Check sheet for the modelled part. Datum: model origin and axes. Units: mm. Face numbers are marked on the shaded views. A direction names the side the tool comes from. Give positions to 0.01 mm unless a question says otherwise; leave off trailing zeros. Order: outer loops, then holes, each group sorted by start corner. A loop starts at its lowest first (then second) coordinate and runs counter-clockwise, first axis right, second up.
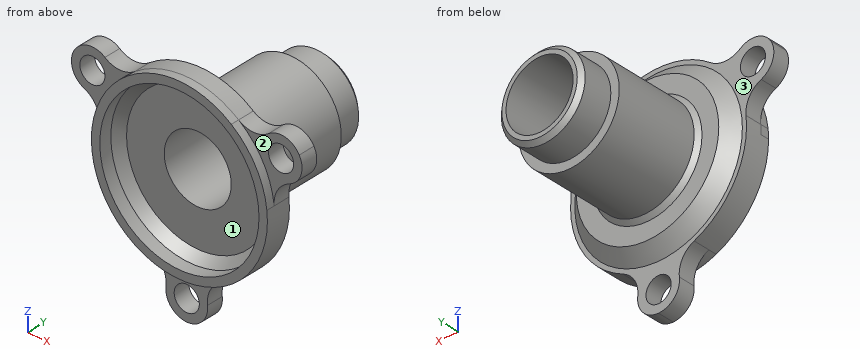
```python
from build123d import *

# Parameters (mm, degrees)
CHAMFER_1_SIZE      = 0.5
SKETCH_2_R          = 1.5
CUT_EXTRUDE_1_DEPTH = 28.256925725


with BuildPart() as part:
    # 草图1 → 旋转1 (revolve)
    with BuildSketch(Plane.XY, mode=Mode.PRIVATE) as revolve_1_sk:
        Polygon((10.5, 0), (15.5, 0), (15.5, 2), (10, 2), (8.5, 3.5), (6, 3.5), (6, 14.2), (5, 14.2), (5, 18.2), (4, 18.2), (4, 1.5), (8.5, 1.5), (9.5, 0.5), (9.5, -1), (10.5, -1), align=None)
    revolve(revolve_1_sk.sketch.rotate(Axis((0, 18.9, 0), (0, -1, 0)), 180), axis=Axis((0, 18.9, 0), (0, -1, 0)))

    # 倒角1
    chamfer_1_edges = [part.edges().sort_by_distance(p)[0] for p in [
        (5, 18.2, 0),
        (6, 3.5, 0),
    ]]
    chamfer(chamfer_1_edges, length=CHAMFER_1_SIZE)

    # 草图2 → 切除-拉伸1 (cut, through all)
    with BuildSketch(Plane(origin=(0, 2, 0), x_dir=(1, 0, 0), z_dir=(0, 1, 0))):
        with Locations(Location((0, 13, 0), (0, 0, 270))):
            Circle(SKETCH_2_R)
        with Locations(Location((11.258330249, -6.5, 0), (0, 0, 270))):
            Circle(SKETCH_2_R)
        with Locations(Location((-11.258330249, -6.5, 0), (0, 0, 270))):
            Circle(SKETCH_2_R)
        with BuildLine():
            ThreePointArc((13.423393657, -7.750000175), (13.423393809, 7.749999912), (0, 15.5))
            ThreePointArc((0, 15.5), (1.86989398, 14.659366296), (2.482271238, 12.702797203))
            ThreePointArc((2.482271238, 12.702797203), (2.853955321, 10.861790304), (4.247441896, 9.602564103))
            ThreePointArc((4.247441896, 9.602564103), (9.09326674, 5.25), (10.439785402, -1.122889469))
            ThreePointArc((10.439785402, -1.122889469), (10.833563994, -2.959297343), (12.242080696, -4.20168865))
            ThreePointArc((12.242080696, -4.20168865), (13.630330638, -5.710307555), (13.423393657, -7.750000175))
        make_face()
        with BuildLine():
            ThreePointArc((-2.482271238, 12.702797203), (-1.86989398, 14.659366296), (0, 15.5))
            ThreePointArc((0, 15.5), (-13.42339379, 7.749999945), (-13.423393696, -7.750000109))
            ThreePointArc((-13.423393696, -7.750000109), (-13.630330625, -5.710307519), (-12.242080696, -4.20168865))
            ThreePointArc((-12.242080696, -4.20168865), (-10.833563994, -2.959297343), (-10.439785402, -1.122889469))
            ThreePointArc((-10.439785402, -1.122889469), (-9.09326674, 5.25), (-4.247441896, 9.602564103))
            ThreePointArc((-4.247441896, 9.602564103), (-2.853955321, 10.861790304), (-2.482271238, 12.702797203))
        make_face()
        with BuildLine():
            ThreePointArc((-13.423393696, -7.750000109), (-3.8e-08, -15.5), (13.423393657, -7.750000175))
            ThreePointArc((13.423393657, -7.750000175), (11.760436526, -8.949058857), (9.759809458, -8.501108552))
            ThreePointArc((9.759809458, -8.501108552), (7.979608673, -7.902492961), (6.192343507, -8.479674634))
            ThreePointArc((6.192343507, -8.479674634), (0, -10.5), (-6.192343507, -8.479674634))
            ThreePointArc((-6.192343507, -8.479674634), (-7.979608673, -7.902492961), (-9.759809458, -8.501108552))
            ThreePointArc((-9.759809458, -8.501108552), (-11.760436564, -8.94905885), (-13.423393696, -7.750000109))
        make_face()
    extrude(amount=-CUT_EXTRUDE_1_DEPTH, mode=Mode.SUBTRACT)


solid = part.part
```
(1) Cross-section at B-B on x = 0.5. Count the separate pieces of the cut face and the enclosed holes in it, then the cut area to 3 significant figures.
Response values:
separate pieces: 3
enclosed holes: 0
area: 83.7 mm2
(2) Material ranges on L1, parallel to X at y = 1.1, z = -13; L2, parallel to Y at x = -8, z = 7.5; L3, parallel to Y at x = 0.25, z = -7, recorded low to high.
Response values:
L1: x = -2.5 to -1.5, 1.5 to 2.5
L2: y = 0 to 2
L3: y = 1.5 to 3.5
(3) Set-up check for the marked faces 1, 2 and 3: record each of +Z, -Z, +X, -X, +Y, -Y from which the full face is reachable in a straight line by a thin tool's end or side.
Response values:
face 1: -Y
face 2: +Z, +X, -Y
face 3: +Y
(4) Gauge pin test, flat ends, axial feed: pin 1 Ø8 at (x, y) = (-3.5, 5) entering from +Z; pin 2 Ø10 at (x, y) = (-7.5, 10.5) entering from -Z; pin 3 Ø2.5 at (x, z) = (11.26, 6.5) entering from +Y; pin 4 Ø10 at (x, y) = (-7, 11) entering from +Z. Record the tip position at first contact, or that the pin passes through.
Response values:
pin 1: stops at z = 10.47
pin 2: stops at z = -5.45
pin 3: passes through
pin 4: stops at z = 5.66
(5) Cross-section at A-A on y = 8.5. Enter the section's corners in (x, z), then the cut area to 3 significant figures.
Response values:
outline: circle Ø12 at (0, 0); hole circle Ø8 at (0, 0)
area: 62.8 mm2
